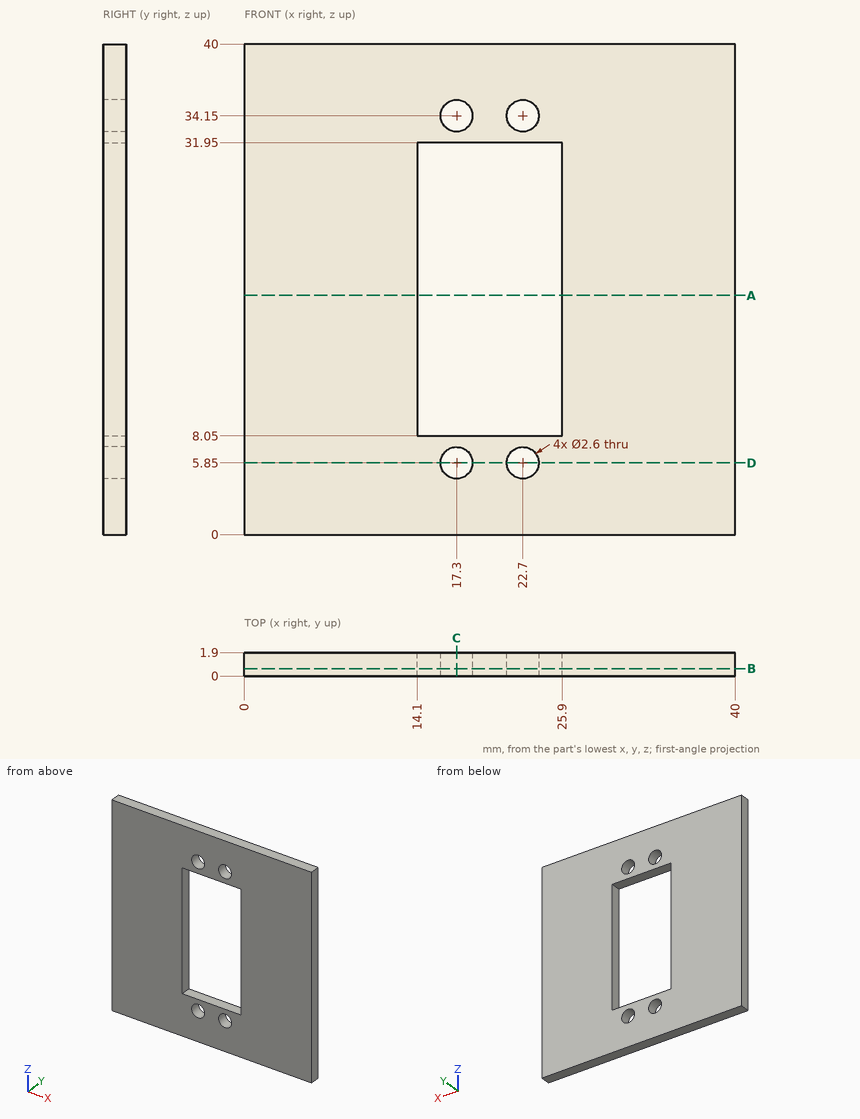
Job drawing, mm, ordinate dimensions from the low corner. One solid piece. Give positions to 0.01 mm unless a question says otherwise; leave off trailing zeros. Loops run counter-clockwise (first coordinate to the right, second up) from the corner with the lowest first, then second, coordinate; pieces in that order, holes last. Notation, with made-up numbers: (67.25, 39) -> (82.25, 39) arc R20 ccw to (82.25, 63) -> close; hole circle Ø1 at (73.25, 74). An arc over 180 degrees is marked (long way). Use a Markdown table: item, result. Add a question column.
(1) Slice it at A-A on z = 19.5. List the corners of the cut face in (x, y).
(2) Slice it at C-C on x = 17.3. List the corners of the cut face in (y, z), and give its area (3 significant figures).
(3) Slice it at D-D on z = 5.85. List the corners of the cut face in (x, y), and give its area (3 significant figures).
(4) Slice it at B-B on y = 0.6. List the corners of the cut face in (x, z).
(5) Wall check: line 1 along Z through (x, y) = (17.3, 1.45); line 2 along X through (y, z) = (0.35, 13); line 3 along Z through (x, y) = (20, 0.75). Give the ranges that are in metal, low to high.
Filled sheet:
| question | item | result |
|---|---|---|
| 1 | outline | (0, 0) -> (14.1, 0) -> (14.1, 1.9) -> (0, 1.9) -> close; (25.9, 0) -> (40, 0) -> (40, 1.9) -> (25.9, 1.9) -> close |
| 2 | outline | (0, 0) -> (1.9, 0) -> (1.9, 4.55) -> (0, 4.55) -> close; (0, 7.15) -> (1.9, 7.15) -> (1.9, 8.05) -> (0, 8.05) -> close; (0, 31.95) -> (1.9, 31.95) -> (1.9, 32.85) -> (0, 32.85) -> close; (0, 35.45) -> (1.9, 35.45) -> (1.9, 40) -> (0, 40) -> close |
| 2 | area | 20.7 mm2 |
| 3 | outline | (0, 0) -> (16, 0) -> (16, 1.9) -> (0, 1.9) -> close; (18.6, 0) -> (21.4, 0) -> (21.4, 1.9) -> (18.6, 1.9) -> close; (24, 0) -> (40, 0) -> (40, 1.9) -> (24, 1.9) -> close |
| 3 | area | 66.1 mm2 |
| 4 | outline | (0, 0) -> (40, 0) -> (40, 40) -> (0, 40) -> close; hole (14.1, 8.05) -> (25.9, 8.05) -> (25.9, 31.95) -> (14.1, 31.95) -> close; hole circle Ø2.6 at (17.3, 5.85); hole circle Ø2.6 at (17.3, 34.15); hole circle Ø2.6 at (22.7, 5.85); hole circle Ø2.6 at (22.7, 34.15) |
| 5 | line 1 | 0 to 4.55, 7.15 to 8.05, 31.95 to 32.85, 35.45 to 40 |
| 5 | line 2 | 0 to 14.1, 25.9 to 40 |
| 5 | line 3 | 0 to 8.05, 31.95 to 40 |
